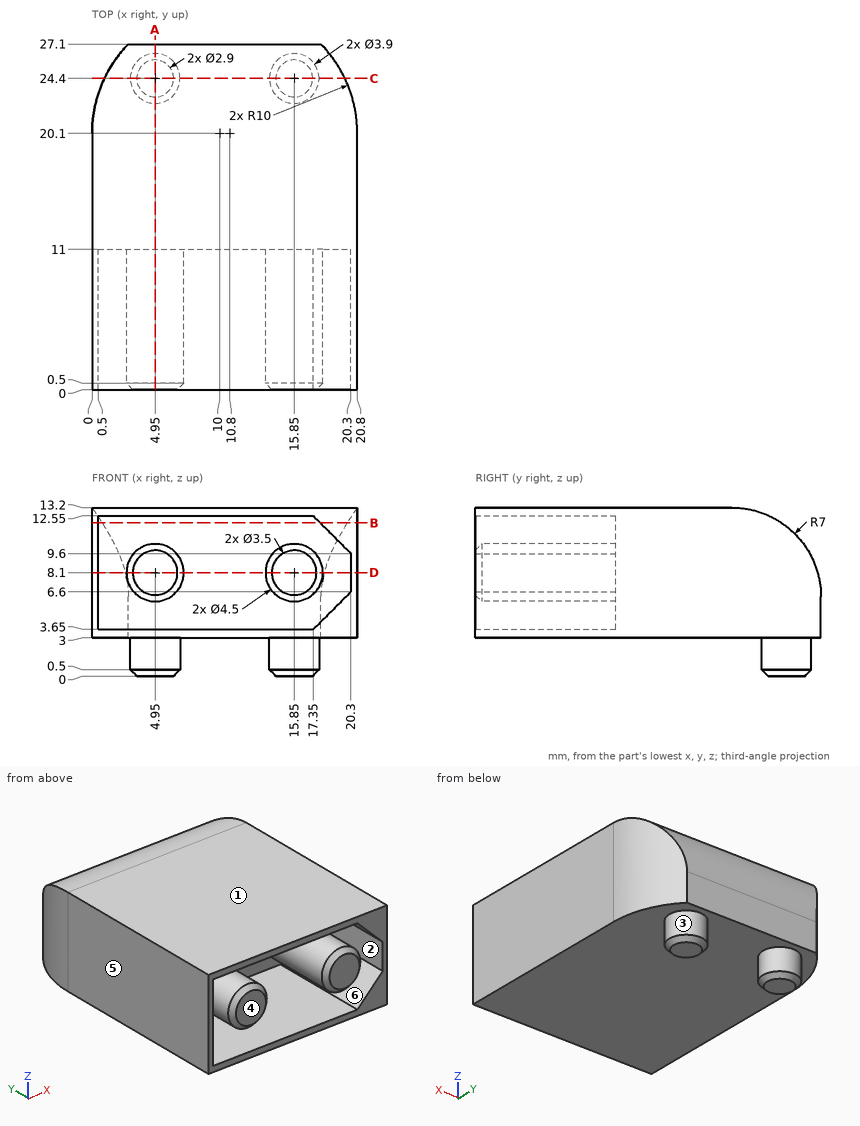
Design review of the part shown in the three views and the two pictorial views. Dimensions are in mm from the part's minimum x, y and z. A direction names the side the tool comes from. Round coordinates to 2 decimals unless told otherwise and drop trailing zeros. Write each loop counter-clockwise with the first axis right and the second up, starting at its lowest first coordinate (ties: lowest second). Pieces come first, ordered by that corner, then holes. Notation, with made-up numbers: (57, 37) - (92, 37) arc R35 cw to (92, 75) - close; hole circle Ø8 at (75.5, -10.5). An arc over 180 degrees is marked (long way). Write item = value, one per line. Start each with the question number.
1. Consider section D-D on z = 8.1. State the section outline as (x, y) points.
2. For pin 1 Ø6 at (x, y) = (10.5, 9.5) entering from -Z; pin 2 Ø3 at (y, z) = (24, 8) entering from -X; pin 3 Ø1.5 at (x, z) = (17.5, 6) entering from -Y, all flat-tipped, find the tip position at first contact; note any pin that passes through.
3. Consider section A-A on x = 4.95. State the section outline as (y, z) points.
4. Consider section B-B on z = 12. State the section outline as (x, y) points, plus the area to 3 significant figures.
5. Consider section C-C on y = 24.4. State the section outline as (x, z) points, plus the area to 3 significant figures.
6. Draft analysis for pull direction X (two halves, no side actions). For the marked faces 4, 5 and 6, state which applies: released by +X, released by -X, zero draft, split by the parting line, or undercut.
7. For the marked faces 1, 2 and 3, list the 3-axis set-ups (+Z, -Z, +X, -X, +Y, -Y) from which the entire face can be reached by the end or side of a thin tool; tool diameter is ignored.
8. Wall thickness on L1, parallel to Z at x = 5, y = 4.5; L2, parallel to Y at x = 6.25, z = 4.5; L3, parallel to Z at x = 15, y = 3.75: over which ranges is each line inside the solid? List them lowest first.
Evaluation:
q1.outline = (0, 0) - (0.5, 0) - (0.5, 11) - (2.7, 11) - (2.7, 0.5) - (3.2, 0) - (6.7, 0) - (7.2, 0.5) - (7.2, 11) - (13.6, 11) - (13.6, 0.5) - (14.1, 0) - (17.6, 0) - (18.1, 0.5) - (18.1, 11) - (20.3, 11) - (20.3, 0) - (20.8, 0) - (20.8, 20.1) arc R10 ccw to (18.19, 26.84) - (2.61, 26.84) arc R10 ccw to (0, 20.1) - close
q2.pin_1 = 3
q2.pin_2 = 0.29
q2.pin_3 = 0.17
q3.outline = (0, 3) - (22.45, 3) - (22.45, 0.5) - (22.95, 0) - (25.85, 0) - (26.35, 0.5) - (26.35, 3) - (27.1, 3) - (27.1, 6.2) arc R7 ccw to (20.1, 13.2) - (0, 13.2) - (0, 12.55) - (11, 12.55) - (11, 10.35) - (0.5, 10.35) - (0, 9.85) - (0, 6.35) - (0.5, 5.85) - (11, 5.85) - (11, 3.65) - (0, 3.65) - close
q4.outline = (0, 0) - (0.5, 0) - (0.5, 11) - (17.9, 11) - (17.9, 0) - (20.8, 0) - (20.8, 20.1) arc R10 ccw to (20, 24.02) - (0.8, 24.02) arc R10 ccw to (0, 20.1) - close
q4.area = 306 mm2
q5.outline = (0.97, 3) - (3, 3) - (3, 0.5) - (3.5, 0) - (6.4, 0) - (6.9, 0.5) - (6.9, 3) - (13.9, 3) - (13.9, 0.5) - (14.4, 0) - (17.3, 0) - (17.8, 0.5) - (17.8, 3) - (19.83, 3) - (19.83, 11.72) - (0.97, 11.72) - close
q5.area = 187 mm2
q6.face_4 = zero draft
q6.face_5 = released by -X
q6.face_6 = undercut
q7.face_1 = +Z, +X, -X, +Y, -Y
q7.face_2 = -Y
q7.face_3 = -Z
q8.L1 = 3 to 3.65, 5.85 to 10.35, 12.55 to 13.2
q8.L2 = 11 to 27.1
q8.L3 = 3 to 3.65, 6.02 to 10.18, 12.55 to 13.2
